For this review, use the dimensioned drawing (mm, ordinates from the lowest corner) and the shaded views. A direction names the side the tool comes from. Round coordinates to 2 decimals unless told otherwise and drop trailing zeros. Write each loop counter-clockwise with the first axis right and the second up, starting at its lowest first coordinate (ties: lowest second). Pieces come first, ordered by that corner, then holes. Notation, with made-up numbers: M 29.5,39.5 L 65.5,39.5 A23 cw 65.5,77.5 Z; hole C 56.25,3.25 d4. An arc over 180 degrees is marked long. Use CSV: the item, a comma, the result in double quotes.
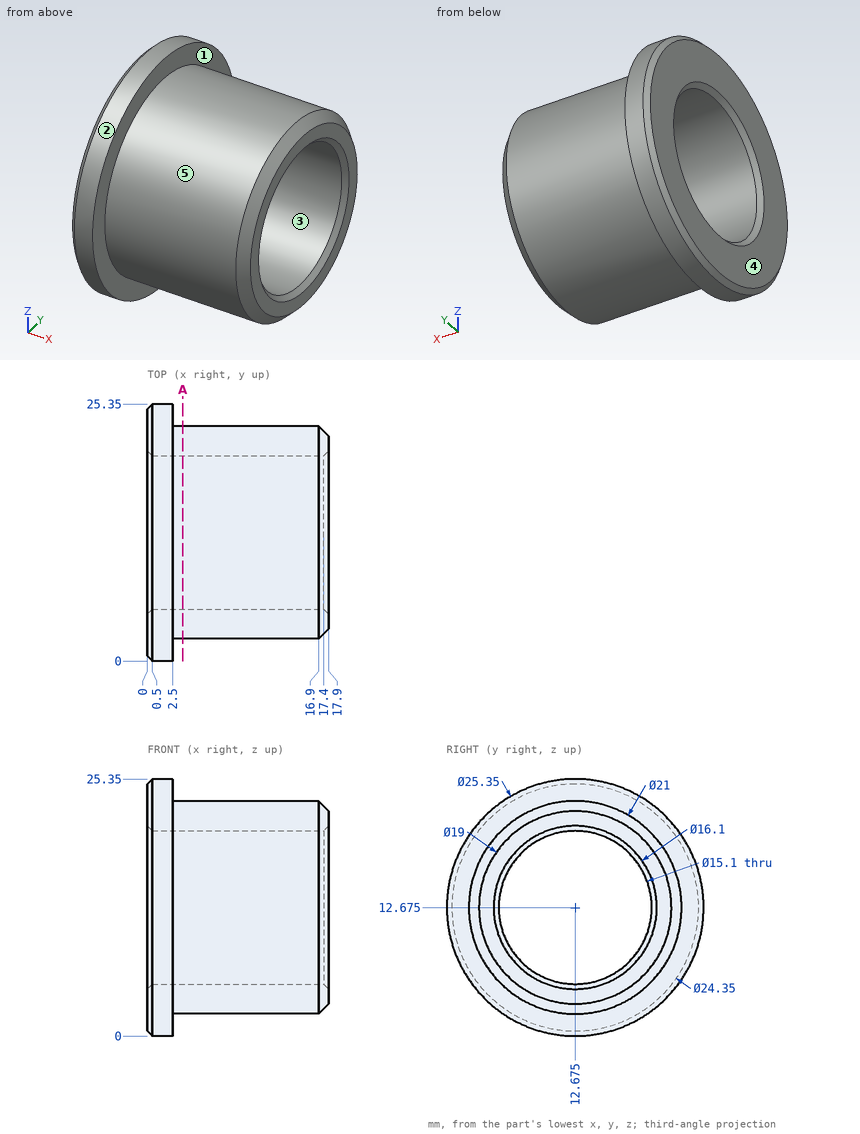
1) Machinability: for the marked faces 1 and 2, which of the approach directions +Z, -Z, +X, -X, +Y, -Y give a long, thin tool a straight path to every point of the face, cutting with its end or side? Answer none if there is none.
Answers:
face 1,"+X"
face 2,"+X, -X"
2) Add section A-A on x = 3.5. Write out the cut boundary in (y, z) (3 decimals), then the cut area to 3 significant figures.
Answers:
outline,"C 12.675,12.675 d21; hole C 12.675,12.675 d15.1"
area,"167 mm²"
3) For pin 1 Ø1.5 at (y, z) = (16.5, 19.5) entering from -X; pin 2 Ø2 at (x, z) = (2.5, 16.5) entering from -Y; pin 3 Ø10 at (x, z) = (11, 16) entering from +Y (3 decimals); pin 4 Ø1 at (x, z) = (3.5, 13.5) entering from -Y, all flat-tipped, find the tip position at first contact; note any pin that passes through.
Answers:
pin 1,"x = 0"
pin 2,"y = 0.32"
pin 3,"y = 23.175"
pin 4,"y = 2.18"
4) The part is to be moulded in two halves that separate along Y. For the marked faces 3, 4 and 5, say which applies: released by +Y, released by -Y, zero draft, split by the parting line, or undercut.
Answers:
face 3,"undercut"
face 4,"zero draft"
face 5,"split by the parting line"
5) Wall thickness on line 1 along Z through (x, y) = (13.25, 13); line 2 along Z through (x, y) = (12, 14.75); line 3 along X through (y, z) = (1.75, 11): over which ranges is each line inside the solid? List them lowest first. Write a range as [from, to].
Answers:
line 1,"[2.18, 5.13], [20.22, 23.17]"
line 2,"[2.38, 5.42], [19.93, 22.97]"
line 3,"[0, 2.5]"
